from build123d import *

# Parameters (mm, degrees)
SKETCH1_W           = 68
SKETCH1_H           = 68
SKETCH1_R           = 2.6
SKETCH1_R_2         = 2.1
SKETCH1_R_3         = 20
BOSS_EXTRUDE1_DEPTH = 3.175
FILLET2_R           = 3


with BuildPart() as part:
    # Sketch1 → Boss-Extrude1 (new, symmetric)
    with BuildSketch(Plane.XY):
        Rectangle(SKETCH1_W, SKETCH1_H)
        with Locations((-23.57, 23.57)):
            Circle(SKETCH1_R, mode=Mode.SUBTRACT)
        with Locations((23.57, 23.57)):
            Circle(SKETCH1_R, mode=Mode.SUBTRACT)
        with Locations((23.57, -23.57)):
            Circle(SKETCH1_R, mode=Mode.SUBTRACT)
        with Locations((-23.57, -23.57)):
            Circle(SKETCH1_R, mode=Mode.SUBTRACT)
        with Locations((-31, 31)):
            Circle(SKETCH1_R_2, mode=Mode.SUBTRACT)
        with Locations((31, 31)):
            Circle(SKETCH1_R_2, mode=Mode.SUBTRACT)
        with Locations((31, -31)):
            Circle(SKETCH1_R_2, mode=Mode.SUBTRACT)
        with Locations((-31, -31)):
            Circle(SKETCH1_R_2, mode=Mode.SUBTRACT)
        Circle(SKETCH1_R_3, mode=Mode.SUBTRACT)
    extrude(amount=BOSS_EXTRUDE1_DEPTH, both=True)

    # Fillet2
    fillet2_edges = [part.edges().sort_by_distance(p)[0] for p in [
        (-34, 34, 0),
        (34, 34, 0),
        (34, -34, 0),
        (-34, -34, 0),
    ]]
    fillet(fillet2_edges, radius=FILLET2_R)


solid = part.part
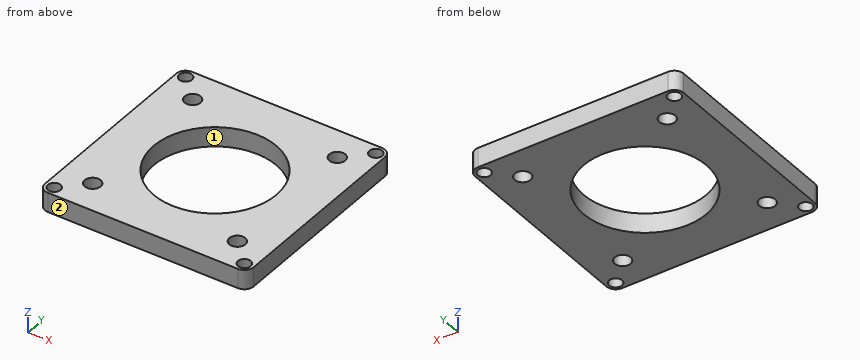
The model under review builds one solid part; all positions refer to its coordinate system, in mm. Face numbers are marked on the shaded views. Round coordinates to 2 decimals unless told otherwise and drop trailing zeros. Order: outer loops, then holes, each group sorted by start corner. A loop starts at its lowest first (then second) coordinate and runs counter-clockwise, first axis right, second up. Notation, with made-up numbers: (41, 4) -> (58, 4) arc R20 cw to (58, 16) -> close; hole circle Ø3 at (1, -20). An arc over 180 degrees is marked (long way). Return JSON: item names as keys, results as strings.
1. Insertion check: P1, Ø6.5, axis at x = -31, y = -31, coming from the +Z side (3 decimals); P2, Ø4.5, axis at x = 23.57, y = 23.57, coming from the -Z side. Each pin has a flat end and moves straight along its axis. Give the tip position at first contact, or say it passes through.
Answer block:
{"P1": "stops at z = 3.175", "P2": "passes through"}
2. Take a section at C-C (y = 0). Write out the cut boundary in (x, z) (3 decimals).
Answer block:
{"outline": "(-34, -3.175) -> (-20, -3.175) -> (-20, 3.175) -> (-34, 3.175) -> close; (20, -3.175) -> (34, -3.175) -> (34, 3.175) -> (20, 3.175) -> close"}
3. Take a section at D-D (x = 10). Write out the cut boundary in (y, z) (1 decimal), then the cut area to 3 significant figures.
Answer block:
{"outline": "(-34, -3.2) -> (-17.3, -3.2) -> (-17.3, 3.2) -> (-34, 3.2) -> close; (17.3, -3.2) -> (34, -3.2) -> (34, 3.2) -> (17.3, 3.2) -> close", "area": "212 mm²"}
4. Take a section at A-A (x = -23.57). Write out the cut boundary in (y, z) (3 decimals), then the cut area to 3 significant figures.
Answer block:
{"outline": "(-34, -3.175) -> (-26.17, -3.175) -> (-26.17, 3.175) -> (-34, 3.175) -> close; (-20.97, -3.175) -> (20.97, -3.175) -> (20.97, 3.175) -> (-20.97, 3.175) -> close; (26.17, -3.175) -> (34, -3.175) -> (34, 3.175) -> (26.17, 3.175) -> close", "area": "366 mm²"}
5. For L1, parallel to Y at x = -23.57, z = 0; L2, parallel to Y at x = 31, z = 0.25; L3, parallel to Y at x = 11, z = -2.25, list the stretches that pass through material, from the lowest coordinate up. Write a range as [from, to].
Answer block:
{"L1": "y = [-34, -26.17], [-20.97, 20.97], [26.17, 34]", "L2": "y = [-34, -33.1], [-28.9, 28.9], [33.1, 34]", "L3": "y = [-34, -16.7], [16.7, 34]"}
6. The part is to be moulded in two halves that separate along X. For the marked faces 1 and 2, say which applies: +X half, -X half, draft (parallel to the pull), parting line (faces both ways), or undercut.
Answer block:
{"face 1": "undercut", "face 2": "draft"}
